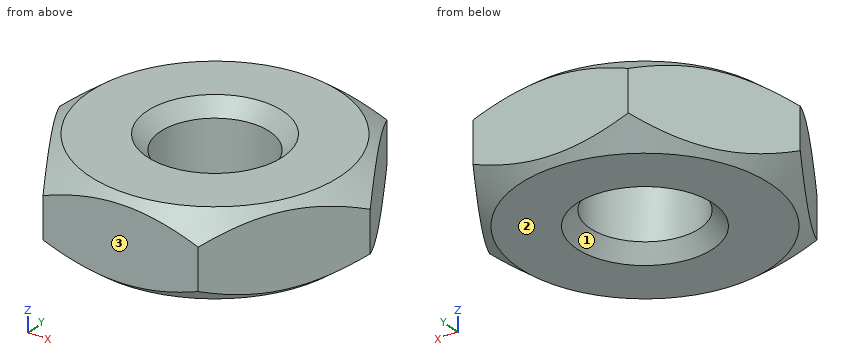
from build123d import *

# Parameters (mm, degrees)
SKETCH1_R      = 1.125
EXTRUDE1_DEPTH = 0.875


with BuildPart() as part:
    # Sketch1 → Extrude1 (new body, symmetric)
    with BuildSketch(Plane.XY):
        Polygon((3.175426481, 0), (1.58771324, 2.75), (-1.58771324, 2.75), (-3.175426481, 0), (-1.58771324, -2.75), (1.58771324, -2.75), align=None)
        Circle(SKETCH1_R, mode=Mode.SUBTRACT)
    extrude(amount=EXTRUDE1_DEPTH, both=True)

    # Sketch2 → Cut-Revolve1 (revolve, cut)
    with BuildSketch(Plane(origin=(0, 0, 0), x_dir=(1, 0, 0), z_dir=(0, 1, 0))):
        Polygon((3.175426481, 0.875), (3.175426481, 0.422248701), (2.579675658, 0.875), align=None)
        Polygon((3.175426481, -0.875), (3.175426481, -0.422248701), (2.579675658, -0.875), align=None)
        Polygon((1.042426481, 0.875), (1.398698822, 0.875), (1.042426481, 0.47968772), align=None)
        Polygon((1.042426481, -0.875), (1.398698822, -0.875), (1.042426481, -0.47968772), align=None)
    revolve(axis=Axis((0, 0, -0.875), (0, 0, 1)), mode=Mode.SUBTRACT)


solid = part.part
The model under review builds one solid part; all positions refer to its coordinate system, in mm. Face numbers are marked on the shaded views. Coordinates: 2 decimals unless noted, no trailing zeros. Loops run counter-clockwise (first coordinate to the right, second up) from the corner with the lowest first, then second, coordinate; pieces in that order, holes last.
(1) Draft analysis for pull direction Y (two halves, no side actions). For the marked faces 1, 2 and 3, state which applies: +Y half, -Y half, draft (parallel to the pull), parting line (faces both ways), or undercut.
Determined:
face 1: undercut
face 2: draft
face 3: -Y half
(2) Consider section B-B, the plane z = 0.25. Give the boundary of the cut face in (x, y) (3 decimals), plus the area to 3 significant figures.
Determined:
outline: (-3.175, 0) - (-1.588, -2.75) - (1.588, -2.75) - (3.175, 0) - (1.588, 2.75) - (-1.588, 2.75) - close; hole circle Ø2.25 at (0, 0)
area: 22.2 mm2
(3) Wall thickness on L1, parallel to Y at x = 0, z = -0.1 (3 decimals); L2, parallel to X at y = -0.2, z = 0.65; L3, parallel to Y at x = 1, z = -0.5: over which ranges is each line inside the solid? List them lowest first.
Determined:
L1: y = -2.75 to -1.125, 1.125 to 2.75
L2: x = -2.87 to -1.18, 1.18 to 2.87
L3: y = -2.75 to -0.52, 0.52 to 2.75
(4) Consider section A-A, the plane x = 0. Give the boundary of the cut face in (y, z) (3 decimals), plus the area to 3 significant figures.
Determined:
outline: (-2.75, -0.746) - (-2.58, -0.875) - (-1.399, -0.875) - (-1.125, -0.571) - (-1.125, 0.571) - (-1.399, 0.875) - (-2.58, 0.875) - (-2.75, 0.746) - close; (1.125, -0.571) - (1.399, -0.875) - (2.58, -0.875) - (2.75, -0.746) - (2.75, 0.746) - (2.58, 0.875) - (1.399, 0.875) - (1.125, 0.571) - close
area: 5.48 mm2
(5) Insertion check: P1, Ø1, axis at x = -1.5, z = 0.5, coming from the -Y side. The pin has a flat end and moves straight along its axis. Give the tip position at first contact, or say it passes through.
Determined:
P1: stops at y = -2.75
(6) Consider section C-C, the plane z = -0.65. Give the boundary of the cut face in (x, y).
Determined:
outline: (-2.8, -0.65) - (-1.96, -2.1) arc R2.88 ccw to (-0.84, -2.75) - (0.84, -2.75) arc R2.88 ccw to (1.96, -2.1) - (2.8, -0.65) arc R2.88 ccw to (2.8, 0.65) - (1.96, 2.1) arc R2.88 ccw to (0.84, 2.75) - (-0.84, 2.75) arc R2.88 ccw to (-1.96, 2.1) - (-2.8, 0.65) arc R2.88 ccw to start; hole circle Ø2.39 at (0, 0)
